```python
from build123d import *

# Parameters (mm, degrees)
BOSS_EXTRUDE2_DEPTH = 88.9
SKETCH8_W           = 5.93725
SKETCH8_H           = 12.7
CUT_EXTRUDE3_DEPTH  = 92.025212307
SKETCH10_W          = 5.93725
SKETCH10_H          = 12.7
CUT_EXTRUDE4_DEPTH  = 92.025212307
SKETCH16_R          = 2.06
CUT_EXTRUDE6_DEPTH  = 2.54


with BuildPart() as part:
    # Sketch4 → Boss-Extrude2 (new body)
    with BuildSketch(Plane(origin=(0, 0, 0), x_dir=(1, 0, 0), z_dir=(0, 1, 0))):
        with BuildLine():
            Line((0, 0), (0, -19.05))
            Line((0, -19.05), (1.016, -19.05))
            Line((1.016, -19.05), (1.016, 0))
            ThreePointArc((1.016, 0), (3.365064987, 0.274963066), (1.143, -0.535060511))
            Line((1.143, -0.535060511), (1.143, -1.933363843))
            ThreePointArc((1.143, -1.933363843), (4.106126962, 1.122980938), (0, 0))
        make_face()
    extrude(amount=BOSS_EXTRUDE2_DEPTH)

    # Sketch8 → Cut-Extrude3 (cut, through all)
    with BuildSketch(Plane(origin=(0, 0, 0), x_dir=(0, 0, -1), z_dir=(1, 0, 0))):
        with Locations((0, 6.35)):
            Rectangle(SKETCH8_W, SKETCH8_H)
        with Locations((0, 31.75)):
            Rectangle(SKETCH8_W, SKETCH8_H)
        with Locations((0, 57.15)):
            Rectangle(SKETCH8_W, SKETCH8_H)
        with Locations((0, 82.55)):
            Rectangle(SKETCH8_W, SKETCH8_H)
    extrude(amount=CUT_EXTRUDE3_DEPTH, mode=Mode.SUBTRACT)

    # Sketch10 → Cut-Extrude4 (cut, through all)
    with BuildSketch(Plane(origin=(0, 0, 0), x_dir=(0, 0, -1), z_dir=(1, 0, 0))):
        with Locations((0, 44.45)):
            Rectangle(SKETCH10_W, SKETCH10_H)
    extrude(amount=CUT_EXTRUDE4_DEPTH, mode=Mode.SUBTRACT)

    # Sketch16 → Cut-Extrude6 (cut)
    with BuildSketch(Plane.ZY):
        with Locations((11.0093125, 54.45)):
            Circle(SKETCH16_R)
        with Locations((11.0093125, 69.449999972)):
            Circle(SKETCH16_R)
        with Locations((11.0093125, 34.45)):
            Circle(SKETCH16_R)
        with Locations((11.0093125, 19.450000028)):
            Circle(SKETCH16_R)
    extrude(amount=-CUT_EXTRUDE6_DEPTH, mode=Mode.SUBTRACT)


solid = part.part
```
Work out the finished part from the listing and answer in its coordinate system (mm). A direction names the side the tool comes from. Coordinates: 2 decimals unless noted, no trailing zeros. Loops run counter-clockwise (first coordinate to the right, second up) from the corner with the lowest first, then second, coordinate; pieces in that order, holes last. Notation, with made-up numbers: (-18.75, 46) - (-13.75, 46) arc R22 cw to (-13.75, 61) - close; hole circle Ø10 at (84.5, 57.25). An arc over 180 degrees is marked (long way). Use a Markdown table: item, result.
Item 1: For faces 4 (the flat face through (1, 12.7, -1)), 5 (the cylindrical face through (0.5, 17.44, 10.56)), 6 (the flat face through (1, 25.4, -1)), determine the directions among +Z, -Z, +X, -X, +Y, -Y from which every point of the face is accessible in a straight line to the end or side of a thin tool.
Evaluation:
| item | result |
|---|---|
| face 4 | -Z, +X, -X, -Y |
| face 5 | +X, -X |
| face 6 | -Z, +X, -X |
Item 2: Find section B-B, the plane z = 9.75. Determine the outline of the cut face in (x, y), and give its area (3 significant figures).
Evaluation:
| item | result |
|---|---|
| outline | (0, 0) - (1.02, 0) - (1.02, 17.82) - (0, 17.82) - close; (0, 21.08) - (1.02, 21.08) - (1.02, 32.82) - (0, 32.82) - close; (0, 36.08) - (1.02, 36.08) - (1.02, 52.82) - (0, 52.82) - close; (0, 56.08) - (1.02, 56.08) - (1.02, 67.82) - (0, 67.82) - close; (0, 71.08) - (1.02, 71.08) - (1.02, 88.9) - (0, 88.9) - close |
| area | 77.1 mm2 |
Item 3: The mould has two halves that part along Y. Classify faces 1 (the flat face through (1, 76.2, -1)), 2 (the cylindrical face through (3.353, 18.961, -0.322)), 3 (the cylindrical face through (0.5, 52.44, 10.56)): +Y half, -Y half, draft (parallel to the pull), parting line (faces both ways), or undercut.
Evaluation:
| item | result |
|---|---|
| face 1 | +Y half |
| face 2 | draft |
| face 3 | undercut |
Item 4: Find section D-D, the plane z = 4.25. Determine the outline of the cut face in (x, y).
Evaluation:
| item | result |
|---|---|
| outline | (0, 0) - (1.02, 0) - (1.02, 88.9) - (0, 88.9) - close |
Item 5: Given pin 1 Ø6.5 at (y, z) = (69.45, 11.01) entering from -X; pin 2 Ø4.5 at (y, z) = (34.45, 11.01) entering from +X; pin 3 Ø2.5 at (x, z) = (2.21, 0) entering from -Y; pin 4 Ø0.8 at (x, y) = (0.5, 79.5) entering from -Z, each flat-ended and moving along its own axis, determine where each tip first touches the part or whether it passes through.
Evaluation:
| item | result |
|---|---|
| pin 1 | stops at x = 0 |
| pin 2 | stops at x = 1.02 |
| pin 3 | stops at y = 12.7 |
| pin 4 | stops at z = 2.97 |
Item 6: Find section A-A, the plane y = 54.45. Determine the outline of the cut face in (x, z), and give its area (3 significant figures).
Evaluation:
| item | result |
|---|---|
| outline | (0, 2.97) - (1.02, 2.97) - (1.02, 8.95) - (0, 8.95) - close; (0, 13.07) - (1.02, 13.07) - (1.02, 19.05) - (0, 19.05) - close |
| area | 12.2 mm2 |
Item 7: Find section C-C, the plane y = 19.45. Determine the outline of the cut face in (x, z).
Evaluation:
| item | result |
|---|---|
| outline | (0, 0) arc R2.21 ccw (long way) to (1.14, 1.93) - (1.14, 0.54) arc R1.19 cw (long way) to (1.02, 0) - (1.02, 8.95) - (0, 8.95) - close; (0, 13.07) - (1.02, 13.07) - (1.02, 19.05) - (0, 19.05) - close |
Item 8: Consider probe 1 along X at (y, z) = (62, 9); probe 2 along Y at (x, z) = (0.8, 2.75); probe 3 along Z at (x, y) = (0.2, 56). Determine where each line is inside the solid, lowest interval first. Write a range as from..to.
Evaluation:
| item | result |
|---|---|
| probe 1 | x = 0..1.02 |
| probe 2 | y = 12.7..25.4, 63.5..76.2 |
| probe 3 | z = 2.97..9.65, 12.37..19.05 |
